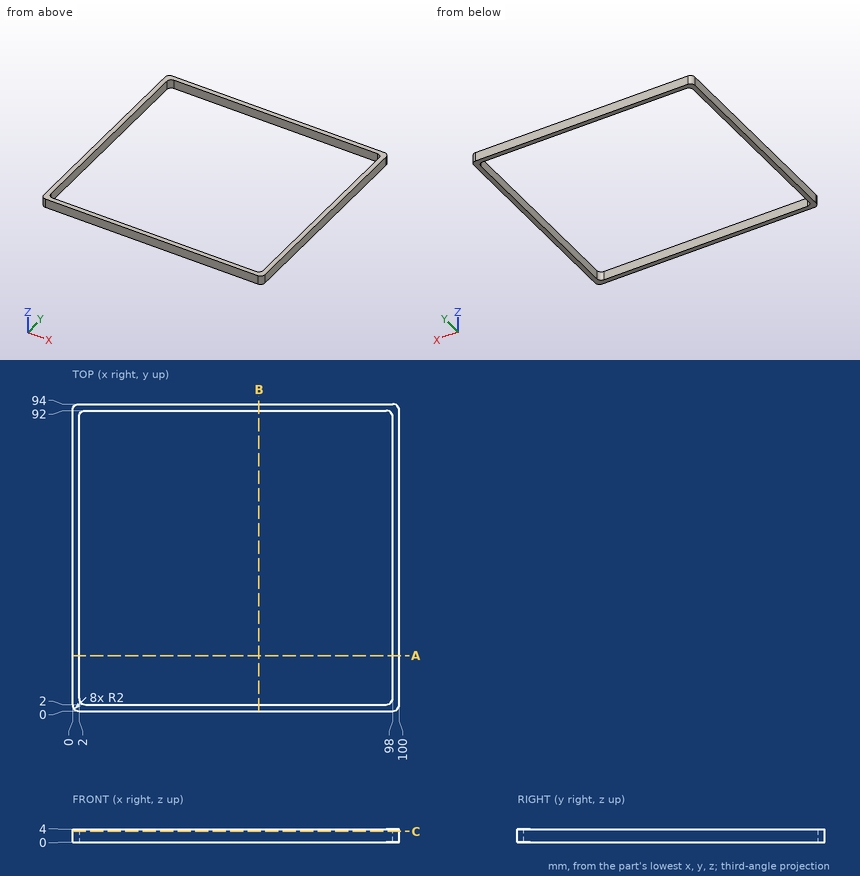
Design review of the part shown in the three views and the two pictorial views. Dimensions are in mm from the part's minimum x, y and z. Give positions to 0.01 mm unless a question says otherwise; leave off trailing zeros. Write each loop counter-clockwise with the first axis right and the second up, starting at its lowest first coordinate (ties: lowest second). Pieces come first, ordered by that corner, then holes.
(1) Add section C-C (z = 3.3). Give the boundary of the cut face in (x, y).
Checked values:
outline: (0, 2) arc R2 ccw to (2, 0) - (98, 0) arc R2 ccw to (100, 2) - (100, 92) arc R2 ccw to (98, 94) - (2, 94) arc R2 ccw to (0, 92) - close; hole (2, 4) arc R2 ccw to (4, 2) - (96, 2) arc R2 ccw to (98, 4) - (98, 90) arc R2 ccw to (96, 92) - (4, 92) arc R2 ccw to (2, 90) - close
(2) Add section B-B (x = 57). Give the boundary of the cut face in (y, z), and give its area (3 significant figures).
Checked values:
outline: (0, 0) - (2, 0) - (2, 4) - (0, 4) - close; (92, 0) - (94, 0) - (94, 4) - (92, 4) - close
area: 16.0 mm2
(3) Wall thickness on line 1 along Y through (x, z) = (25.5, 1.9); line 2 along X through (y, z) = (19, 2.4): over which ranges is each line inside the solid? List them lowest first.
Checked values:
line 1: y = 0 to 2, 92 to 94
line 2: x = 0 to 2, 98 to 100
(4) Add section A-A (y = 17). Give the boundary of the cut face in (x, z), and give its area (3 significant figures).
Checked values:
outline: (0, 0) - (2, 0) - (2, 4) - (0, 4) - close; (98, 0) - (100, 0) - (100, 4) - (98, 4) - close
area: 16.0 mm2
